Drawing for the job (mm, zero at the part's lowest x, y, z). A direction names the side the tool comes from. Round coordinates to 2 decimals unless told otherwise and drop trailing zeros. Order: outer loops, then holes, each group sorted by start corner. A loop starts at its lowest first (then second) coordinate and runs counter-clockwise, first axis right, second up. Notation, with made-up numbers: (59.5, 2) - (69.5, 2) arc R35 cw to (69.5, 41) - close; hole circle Ø10 at (58.25, 26). An arc over 180 degrees is marked (long way). Answer as a JSON object with one key per item and string values.
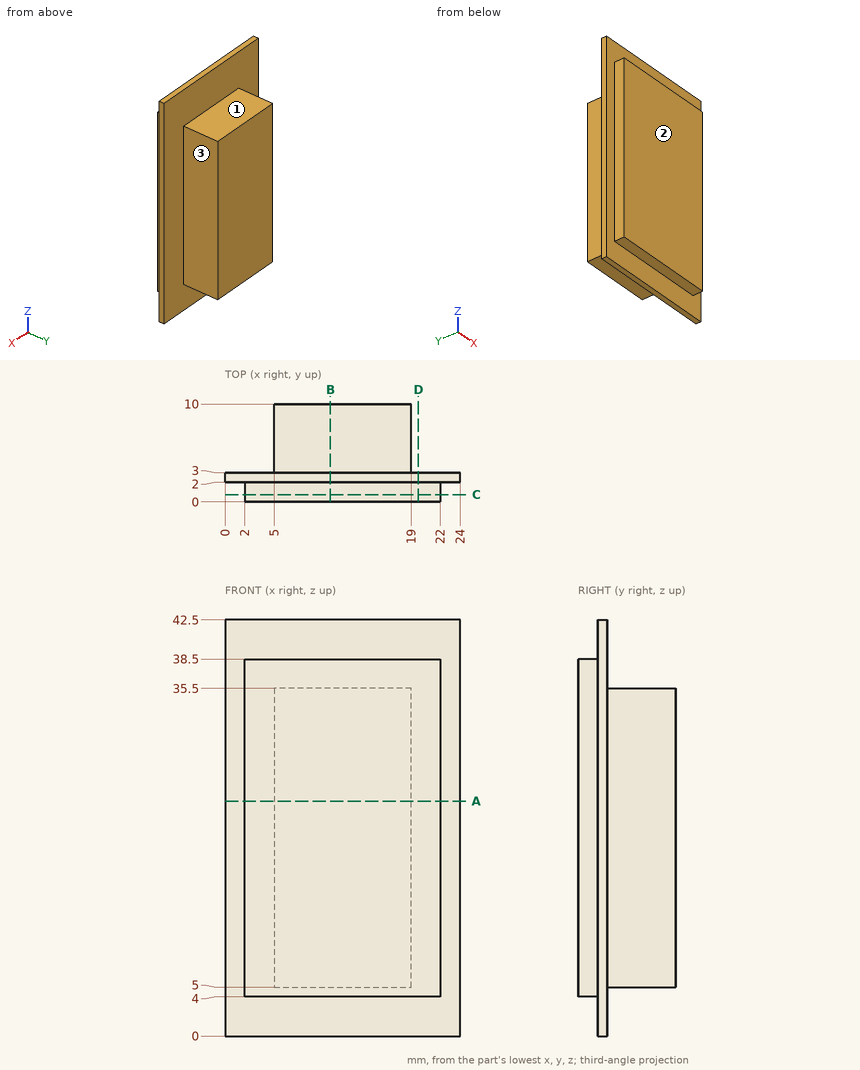
Item 1: Probe L1, parallel to X at y = 9, z = 15.5; L2, parallel to Y at x = 1.75, z = 40.5; L3, parallel to Y at x = 4.25, z = 6. List the from-to ranges inside material, lowest first. Write a range as from..to.
Taken from the geometry:
{"L1": "5..19", "L2": "2..3", "L3": "0..3"}
Item 2: Cut at A-A (z = 24). Write the cut outline in (x, y), plus the area to 3 significant figures.
Taken from the geometry:
{"outline": "(0, 2) - (2, 2) - (2, 0) - (22, 0) - (22, 2) - (24, 2) - (24, 3) - (19, 3) - (19, 10) - (5, 10) - (5, 3) - (0, 3) - close", "area": "162 mm2"}
Item 3: Tool access for the marked faces 1, 2 and 3: list every direction of +Z, -Z, +X, -X, +Y, -Y with a clear straight run to the whole face (end or side of a thin tool).
Taken from the geometry:
{"face 1": "+Z, +X, -X, +Y", "face 2": "+Z, -Z, +X, -X, -Y", "face 3": "+Z, -Z, +X, +Y"}
Item 4: Cut at B-B (x = 10.75). Write the cut outline in (y, z).
Taken from the geometry:
{"outline": "(0, 4) - (2, 4) - (2, 0) - (3, 0) - (3, 5) - (10, 5) - (10, 35.5) - (3, 35.5) - (3, 42.5) - (2, 42.5) - (2, 38.5) - (0, 38.5) - close"}
Item 5: Cut at D-D (x = 19.75). Write the cut outline in (y, z).
Taken from the geometry:
{"outline": "(0, 4) - (2, 4) - (2, 0) - (3, 0) - (3, 42.5) - (2, 42.5) - (2, 38.5) - (0, 38.5) - close"}
Item 6: Drop flat-ended pins along their axis: P1, Ø2, axis at x = 9, y = 0.5, coming from the -Z side; P2, Ø3.5, axis at y = 8, z = 23.5, coming from the +X side; P3, Ø5, axis at y = 1.5, z = 34, coming from the -X side; P4, Ø1.6, axis at y = 0.5, z = 16, coming from the +X side. Give the stop position or say it passes through.
Taken from the geometry:
{"P1": "z = 4", "P2": "x = 19", "P3": "x = 0", "P4": "x = 22"}
Item 7: Cut at C-C (y = 0.75). Write the cut outline in (x, z).
Taken from the geometry:
{"outline": "(2, 4) - (22, 4) - (22, 38.5) - (2, 38.5) - close"}
